For this review, take the finished solid that the model builds, in its own axes (mm). Face numbers are marked on the shaded views. A direction names the side the tool comes from. Round coordinates to 2 decimals unless told otherwise and drop trailing zeros. Loops run counter-clockwise (first coordinate to the right, second up) from the corner with the lowest first, then second, coordinate; pieces in that order, holes last. Notation, with made-up numbers: (64.5, -6) -> (114.5, -6) arc R14 cw to (114.5, 17) -> close; hole circle Ø8 at (-4.5, 48). An arc over 180 degrees is marked (long way). One line per question, with ' | ' between items. Start each with the question number.
1. Consider section C-C (z = 18). Write out the cut boundary in (x, y), and give its area (3 significant figures).
2. For the marked faces 1, 2 and 3, list the 3-axis set-ups (+Z, -Z, +X, -X, +Y, -Y) from which the entire face can be reached by the end or side of a thin tool; tool diameter is ignored.
3. Wall thickness on line 1 along X through (y, z) = (12, 23); line 2 along Z through (x, y) = (22, 40); line 3 along Y through (x, z) = (-12.5, 28): over which ranges is each line inside the solid? List them lowest first.
4. Consider section D-D (y = 57.5). Write out the cut boundary in (x, z).
5. Consider section A-A (y = 0). Write out the cut boundary in (x, z), and give its area (3 significant figures).
6. For pin 1 Ø7.5 at (x, z) = (8, 23) entering from +Y; pin 2 Ø12 at (y, z) = (-24, 28) entering from +X; pin 3 Ø12.5 at (x, z) = (-4, 22.5) entering from -Y, all flat-tipped, find the tip position at first contact; note any pin that passes through.
7. Consider section B-B (x = 0). Write out the cut boundary in (y, z).
```python
from build123d import *

# Parameters (mm, degrees)
F0_R     = 72.029684
F1_DEPTH = 10
F2_W     = 63.849527
F2_H     = 58.85705
F3_DEPTH = 25.4


with BuildPart() as f1:
    # F0 (on Top) → F1 (new body)
    with BuildSketch(Plane.XY):
        Circle(F0_R)
    extrude(amount=F1_DEPTH)

    # F2 (on face) → F3 (join)
    with BuildSketch(Plane.XY.offset(10)):
        with Locations((7.703924, 1.189869)):
            Rectangle(F2_W, F2_H)
    extrude(amount=F3_DEPTH)


solid = f1.part
```
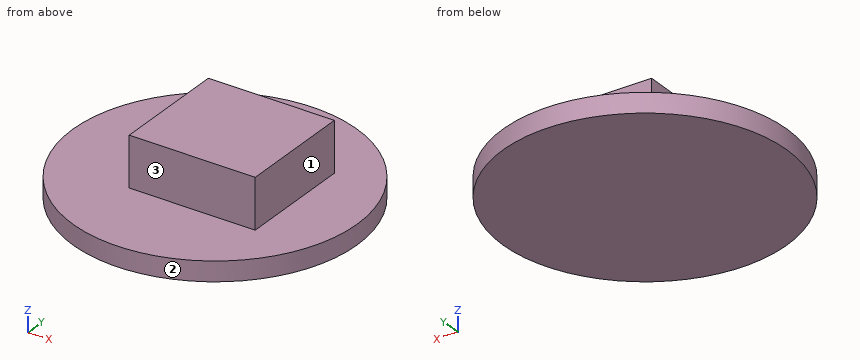
Answer block:
1) outline: (-24.22, -28.24) -> (39.63, -28.24) -> (39.63, 30.62) -> (-24.22, 30.62) -> close | area: 3,760 mm2
2) face 1: +Z, +X, +Y, -Y | face 2: +Z, -Z | face 3: +Z, +X, -X, -Y
3) line 1: x = -24.22 to 39.63 | line 2: z = 0 to 10 | line 3: y = -28.24 to 30.62
4) outline: (-43.38, 0) -> (43.38, 0) -> (43.38, 10) -> (-43.38, 10) -> close
5) outline: (-72.03, 0) -> (72.03, 0) -> (72.03, 10) -> (39.63, 10) -> (39.63, 35.4) -> (-24.22, 35.4) -> (-24.22, 10) -> (-72.03, 10) -> close | area: 3,060 mm2
6) pin 1: stops at y = 30.62 | pin 2: stops at x = 39.63 | pin 3: stops at y = -28.24
7) outline: (-72.03, 0) -> (72.03, 0) -> (72.03, 10) -> (30.62, 10) -> (30.62, 35.4) -> (-28.24, 35.4) -> (-28.24, 10) -> (-72.03, 10) -> close
